```python
from build123d import *

# Parameters (mm, degrees)
SKETCH1_W           = 121
SKETCH1_H           = 121
SKETCH1_W_2         = 115.5
SKETCH1_H_2         = 115.5
BOSS_EXTRUDE1_DEPTH = 55
SKETCH2_W           = 121
SKETCH2_H           = 121
BOSS_EXTRUDE2_DEPTH = 3
FILLET1_R           = 3
FILLET2_R           = 3
SKETCH3_W           = 20
SKETCH3_H           = 10
CUT_EXTRUDE1_DEPTH  = 177
FILLET3_R           = 2.5
FILLET4_R           = 2.5


with BuildPart() as part:
    # Sketch1 → Boss-Extrude1 (new body)
    with BuildSketch(Plane.XY):
        Rectangle(SKETCH1_W, SKETCH1_H)
        Rectangle(SKETCH1_W_2, SKETCH1_H_2, mode=Mode.SUBTRACT)
    extrude(amount=BOSS_EXTRUDE1_DEPTH)

    # Sketch2 → Boss-Extrude2 (add)
    with BuildSketch(Plane.XY.offset(55)):
        Rectangle(SKETCH2_W, SKETCH2_H)
    extrude(amount=BOSS_EXTRUDE2_DEPTH)

    # Fillet1
    fillet1_edges = [part.edges().sort_by_distance(p)[0] for p in [
        (-57.75, 57.75, 27.5),
        (-57.75, -57.75, 27.5),
        (57.75, -57.75, 27.5),
        (57.75, 57.75, 27.5),
        (-57.75, 0, 55),
        (0, -57.75, 55),
        (57.75, 0, 55),
        (0, 57.75, 55),
    ]]
    fillet(fillet1_edges, radius=FILLET1_R)

    # Fillet2
    fillet2_edges = [part.edges().sort_by_distance(p)[0] for p in [
        (-60.5, 0, 58),
        (0, -60.5, 58),
        (60.5, 0, 58),
        (0, 60.5, 58),
        (-60.5, 60.5, 29),
        (60.5, 60.5, 29),
        (60.5, -60.5, 29),
        (-60.5, -60.5, 29),
    ]]
    fillet(fillet2_edges, radius=FILLET2_R)

    # Sketch3 → Cut-Extrude1 (cut)
    with BuildSketch(Plane.XZ.offset(60.5)):
        with Locations((0.054250772, 0.496011987)):
            Rectangle(SKETCH3_W, SKETCH3_H)
    extrude(amount=-CUT_EXTRUDE1_DEPTH, mode=Mode.SUBTRACT)

    # Fillet3
    fillet3_edges = [part.edges().sort_by_distance(p)[0] for p in [
        (-9.945749228, -59.125, 0),
        (-9.945749228, -59.125, 5.496011987),
        (10.054250772, -59.125, 0),
        (10.054250772, -59.125, 5.496011987),
    ]]
    fillet(fillet3_edges, radius=FILLET3_R)

    # Fillet4
    fillet4_edges = [part.edges().sort_by_distance(p)[0] for p in [
        (-9.945749228, 59.125, 0),
        (-9.945749228, 59.125, 5.496011987),
        (10.054250772, 59.125, 0),
        (10.054250772, 59.125, 5.496011987),
    ]]
    fillet(fillet4_edges, radius=FILLET4_R)


solid = part.part
```
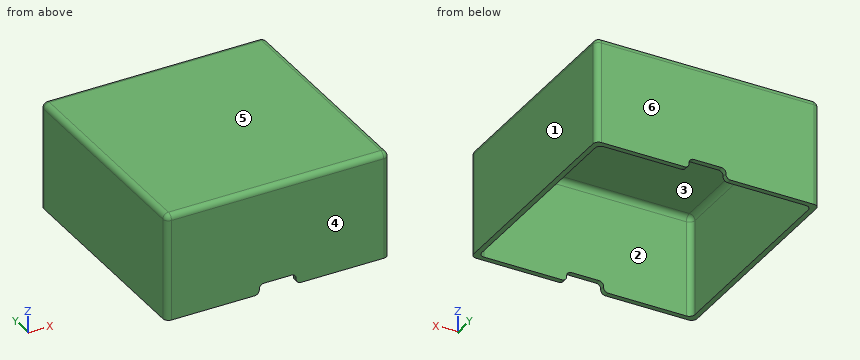
Work out the finished part from the listing and answer in its coordinate system (mm). Face numbers are marked on the shaded views. A direction names the side the tool comes from. Give positions to 0.01 mm unless a question says otherwise; leave off trailing zeros. Loops run counter-clockwise (first coordinate to the right, second up) from the corner with the lowest first, then second, coordinate; pieces in that order, holes last. Notation, with made-up numbers: (-2, 41.5) -> (48, 41.5) arc R26 cw to (48, 73.5) -> close; hole circle Ø11 at (55, -18.5). An arc over 180 degrees is marked (long way). Write item = value, one per line. Start each with the question number.
(1) The mould has two halves that part along Y. Classify the marked faces 3, 4, 5 and 6: +Y half, -Y half, draft (parallel to the pull), parting line (faces both ways), or undercut.
(2) Which of the six approach directions +Z, -Z, +X, -X, +Y, -Y give full straight-line access (tool end or side, diameter ignored) to the marked faces 1 and 2?
(3) Given pin 1 Ø2 at (x, y) = (0, -59.5) entering from -Z; pin 2 Ø4 at (x, y) = (-6, -34) entering from -Z, each flat-ended and moving along its own axis, determine where each tip first touches the part or whether it passes through.
(4) Find section B-B on x = 2.5. Give the vertices of the cut face in (y, z), and give its area (3 significant figures).
(5) Find the intervals of material crossed by probe 1 along X at (y, z) = (26, 16); probe 2 along Z at (x, y) = (-13.5, -51), in increasing order. Write a range as from..to.
(6) Find section A-A on z = 12. Give the vertices of the cut face in (x, y), and give its area (3 significant figures).
(7) Find section C-C on y = -24. Give the vertices of the cut face in (x, z), and give its area (4 significant figures).
From the geometry:
q1.face_3 = undercut
q1.face_4 = -Y half
q1.face_5 = draft
q1.face_6 = +Y half
q2.face_1 = +Z, -Z, +X, +Y, -Y
q2.face_2 = -Z
q3.pin_1 = 5.5
q3.pin_2 = 55
q4.outline = (-60.5, 5.5) -> (-57.75, 5.5) -> (-57.75, 52) arc R3 cw to (-54.75, 55) -> (54.75, 55) arc R3 cw to (57.75, 52) -> (57.75, 5.5) -> (60.5, 5.5) -> (60.5, 55) arc R3 ccw to (57.5, 58) -> (-57.5, 58) arc R3 ccw to (-60.5, 55) -> close
q4.area = 635 mm^2
q5.probe_1 = -60.5..-57.75, 57.75..60.5
q5.probe_2 = 55..58
q6.outline = (-60.5, -57.5) arc R3 ccw to (-57.5, -60.5) -> (57.5, -60.5) arc R3 ccw to (60.5, -57.5) -> (60.5, 57.5) arc R3 ccw to (57.5, 60.5) -> (-57.5, 60.5) arc R3 ccw to (-60.5, 57.5) -> close; hole (-57.75, -54.75) arc R3 ccw to (-54.75, -57.75) -> (54.75, -57.75) arc R3 ccw to (57.75, -54.75) -> (57.75, 54.75) arc R3 ccw to (54.75, 57.75) -> (-54.75, 57.75) arc R3 ccw to (-57.75, 54.75) -> close
q6.area = 1,300 mm^2
q7.outline = (-60.5, 0) -> (-57.75, 0) -> (-57.75, 52) arc R3 cw to (-54.75, 55) -> (54.75, 55) arc R3 cw to (57.75, 52) -> (57.75, 0) -> (60.5, 0) -> (60.5, 55) arc R3 ccw to (57.5, 58) -> (-57.5, 58) arc R3 ccw to (-60.5, 55) -> close
q7.area = 665.5 mm^2
